Verification items for the finished model (mm, model axes). Face numbers are marked on the shaded views. A direction names the side the tool comes from. Round coordinates to 2 decimals unless told otherwise and drop trailing zeros. Write each loop counter-clockwise with the first axis right and the second up, starting at its lowest first coordinate (ties: lowest second). Pieces come first, ordered by that corner, then holes.
from build123d import *

# Parameters (mm, degrees)
F0_W      = 88.9
F0_H      = 50.8
F1_DEPTH  = 38.1
F3_DEPTH  = 38.101
F5_DEPTH  = 25.4
F7_R      = 8.89
F8_DEPTH  = 25.4
F9_W      = 12.7052063286
F9_H      = 2.550378209
F10_DEPTH = 207.518
F11_F1_R  = 25.4
F11_F2_R  = 25.4
F12_W     = 88.9
F12_H     = 12.7
F13_DEPTH = 56.642
F14_R     = 5.08
F15_DEPTH = 1.27


with BuildPart() as f1:
    # F0 (on Front) → F1 (new body)
    with BuildSketch(Plane.XZ):
        with Locations((44.45, 25.4)):
            Rectangle(F0_W, F0_H)
    extrude(amount=F1_DEPTH)

    # F2 (on face) → F3 (cut, through all)
    with BuildSketch(Plane.XZ.offset(38.1)):
        with BuildLine():
            ThreePointArc((9.525, 50.8), (19.7542956671, 26.1042956671), (44.45, 15.875))
            Line((44.45, 15.875), (44.45, 50.8))
            Line((44.45, 50.8), (9.525, 50.8))
        make_face()
        with BuildLine():
            Line((44.45, 50.8), (44.45, 15.875))
            ThreePointArc((44.45, 15.875), (69.1457043329, 26.1042956671), (79.375, 50.8))
            Line((79.375, 50.8), (44.45, 50.8))
        make_face()
    extrude(amount=-F3_DEPTH, mode=Mode.SUBTRACT)

    # F4 (on face) → F5 (cut)
    with BuildSketch(Plane(origin=(0, 0, 0), x_dir=(1, 0, 0), z_dir=(0, 0, -1))):
        with BuildLine():
            ThreePointArc((47.8282, 26.035), (46.8387481282, 28.4237481282), (44.45, 29.4132))
            ThreePointArc((44.45, 29.4132), (42.0612518718, 23.6462518718), (47.8282, 26.035))
        make_face()
    extrude(amount=-F5_DEPTH, mode=Mode.SUBTRACT)

    # F7 (on offset) → F8 (cut)
    with BuildSketch(Plane.XY.offset(9.525)):
        with Locations((44.45, -26.035)):
            Circle(F7_R)
    extrude(amount=F8_DEPTH, mode=Mode.SUBTRACT)

    # F9 (on face) → F10 (cut)
    with BuildSketch(Plane.YZ.offset(88.9)):
        with Locations((-12.7026031643, 1.2751891045)):
            Rectangle(F9_W, F9_H)
    extrude(amount=-F10_DEPTH, mode=Mode.SUBTRACT)

    # F11: fillet of radius 25.4 on 4 edges, made by hand

    # F11_f1
    f11_f1_edges = [f1.edges().sort_by_distance(p)[0] for p in [
        (0, -3.175, 0),
    ]]
    fillet(f11_f1_edges, radius=F11_F1_R)

    # F11_f2
    f11_f2_edges = [f1.edges().sort_by_distance(p)[0] for p in [
        (88.9, -3.175, 0),
    ]]
    fillet(f11_f2_edges, radius=F11_F2_R)

    # F12 (on face) → F13 (cut)
    with BuildSketch(Plane(origin=(0, 0, 0), x_dir=(-1, 0, 0), z_dir=(0, 1, 0))):
        with Locations((-44.45, 44.45)):
            Rectangle(F12_W, F12_H)
    extrude(amount=-F13_DEPTH, mode=Mode.SUBTRACT)

    # F14
    f14_edges = [f1.edges().sort_by_distance(p)[0] for p in [
        (0, -19.05, 38.1),
        (88.9, -19.05, 38.1),
        (7.439488, -38.1, 7.439488),
        (7.439488, 0, 7.439488),
        (5.957966, -38.1, 38.1),
        (82.942034, -38.1, 38.1),
        (5.957966, 0, 38.1),
        (82.942034, 0, 38.1),
    ]]
    fillet(f14_edges, radius=F14_R)

    # F15 (cut): a face of the model
    f15_faces = [f1.faces().sort_by_distance(p)[0] for p in [
        (35.8114471714, -26.035, 9.525),
    ]]
    extrude(f15_faces, amount=-F15_DEPTH, mode=Mode.SUBTRACT)


solid = f1.part
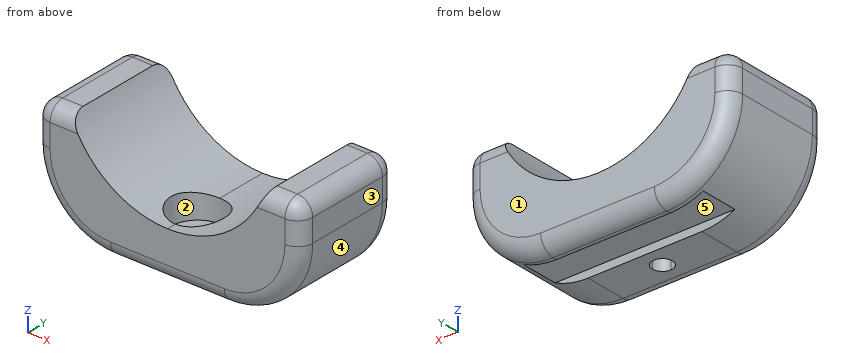
Q1. Depth check by flat-ended pin: P1, Ø8, axis at x = 63.5, z = 22, coming from the -Y side; P2, Ø5, axis at y = -25, z = 13.5, coming from the +X side; P3, Ø14, axis at x = 43.5, y = -26, coming from the +Z side (3 decimals); P4, Ø2, axis at x = 45.5, z = 1, coming from the +Y side. Enter the tip coordinate at first touch or a pass-through.
Recorded:
P1: stops at y = -38.1
P2: stops at x = 87.1
P3: stops at z = 8.255
P4: stops at y = -1.04
Q2. Tool access check on the marked faces 4 and 5. Record the directions out of +Z, -Z, +X, -X, +Y, -Y that give a thin tool (end or side, any length) a straight path to the whole face; none if there is none.
Recorded:
face 4: -Z, +X, +Y, -Y
face 5: -Z, +X, -X
Q3. Sectioned sample at A-A (y = -27.5). Enter the section's corners in (x, z) (3 decimals).
Recorded:
outline: (0, 25.4) arc R25.4 ccw to (25.4, 0) - (41.406, 0) - (41.406, 8.255) - (35.682, 8.255) - (35.682, 16.994) arc R34.925 cw to (11.916, 38.1) - (5.08, 38.1) arc R5.08 ccw to (0, 33.02) - close; (47.494, 0) - (63.5, 0) arc R25.4 ccw to (88.9, 25.4) - (88.9, 33.02) arc R5.08 ccw to (83.82, 38.1) - (76.984, 38.1) arc R34.925 cw to (53.218, 16.994) - (53.218, 8.255) - (47.494, 8.255) - close
Q4. Sectioned sample at D-D (x = 56.5). Enter the section's corners in (y, z), plus the area to 3 significant figures.
Recorded:
outline: (-38.1, 5.08) arc R5.08 ccw to (-33.02, 0) - (-19.06, 0) - (-19.06, 2.55) - (-6.35, 2.55) - (-6.35, 0) - (-5.08, 0) arc R5.08 ccw to (0, 5.08) - (0, 18.02) - (-38.1, 18.02) - close
area: 643 mm2
Q5. Release check for a two-part mould opening along Y. For the marked faces 1, 2 and 3 record: released by +Y, released by -Y, zero draft, split by the parting line, or undercut.
Recorded:
face 1: released by +Y
face 2: undercut
face 3: zero draft
Q6. Sectioned sample at B-B (z = 29). Enter the section's corners in (x, y).
Recorded:
outline: (0, -33.02) arc R5.08 ccw to (5.08, -38.1) - (17.16, -38.1) - (17.16, 0) - (5.08, 0) arc R5.08 ccw to (0, -5.08) - close; (71.74, -38.1) - (83.82, -38.1) arc R5.08 ccw to (88.9, -33.02) - (88.9, -5.08) arc R5.08 ccw to (83.82, 0) - (71.74, 0) - close
Q7. Material ranges on line 1 along Y through (x, z) = (44.45, 4.75); line 2 along X through (y, z) = (-27, 33); line 3 along Y through (x, z) = (44, 15), recorded low to high.
Recorded:
line 1: y = -38.09 to -29.41, -22.66 to -0.01
line 2: x = 0 to 14.4, 74.5 to 88.9
line 3: y = -38.1 to -34.91, -17.16 to 0
